Part print with two shaded views. Sizes in mm from the minimum x, y, z corner. A direction names the side the tool comes from. Round coordinates to 2 decimals unless told otherwise and drop trailing zeros. Write each loop counter-clockwise with the first axis right and the second up, starting at its lowest first coordinate (ties: lowest second). Pieces come first, ordered by that corner, then holes. Notation, with made-up numbers: (22.5, 2.5) -> (72.5, 2.5) arc R25 ccw to (72.5, 29.5) -> close; hole circle Ø2 at (-29, 22). An arc over 180 degrees is marked (long way). Return JSON: item names as keys, results as strings. Group by question number.
(1) Drill centre lines: L1, parallel to Y at x = 20, z = 11.7; L2, parallel to X at y = 8.75, z = 15; L3, parallel to Z at x = 18, y = 19. Where is each one in solid material? Low to high. Write a range as from..to.
(2) Drop flat-ended pins along their axis: pin 1 Ø6.5 at (x, y) = (20, 12.5) entering from +Z; pin 2 Ø13 at (x, y) = (18.5, 14.5) entering from +Z; pin 3 Ø10 at (x, z) = (8.5, 7) entering from +Y; pin 4 Ø8 at (x, y) = (20, 0.5) entering from -Z. Give the stop position or say it passes through.
(3) Mould opens along X. For the marked faces 5, 6, 7 and 8 say: +X half, -X half, draft (parallel to the pull), parting line (faces both ways), or undercut.
(4) Saw through at A-A (z = 8.5). List the corners of the cut face in (x, y), plus the area to 3 significant figures.
(5) Saw through at D-D (y = 8.75). List the corners of the cut face in (x, z), plus the area to 4 significant figures.
(6) Tool access for the marked faces 1, 2, 3 and 4: list every direction of +Z, -Z, +X, -X, +Y, -Y with a clear straight run to the whole face (end or side of a thin tool).
(7) Saw through at B-B (x = 20). List the corners of the cut face in (y, z).
(8) Saw through at C-C (y = 2.5). List the corners of the cut face in (x, z), plus the area to 4 significant figures.
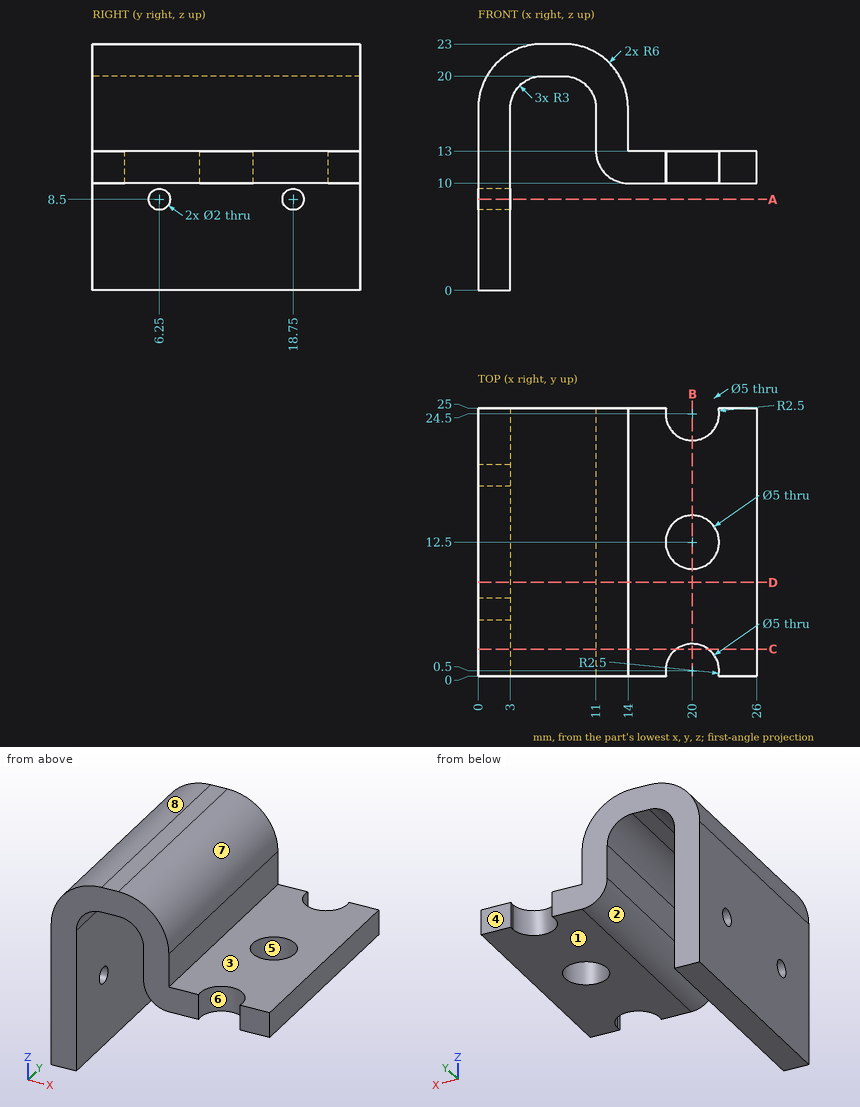
Computed values:
{
 "1": {"L1": "3..10, 15..22", "L2": "0..3, 11..14", "L3": "10..13"},
 "2": {"pin 1": "z = 13", "pin 2": "z = 21.47", "pin 3": "through", "pin 4": "z = 10"},
 "3": {"face 5": "undercut", "face 6": "undercut", "face 7": "+X half", "face 8": "-X half"},
 "4": {"outline": "(0, 0) -> (3, 0) -> (3, 5.25) -> (0, 5.25) -> close; (0, 7.25) -> (3, 7.25) -> (3, 17.75) -> (0, 17.75) -> close; (0, 19.75) -> (3, 19.75) -> (3, 25) -> (0, 25) -> close", "area": "63.0 mm2"},
 "5": {"outline": "(0, 0) -> (3, 0) -> (3, 17) arc R3 cw to (6, 20) -> (8, 20) arc R3 cw to (11, 17) -> (11, 13) arc R3 ccw to (14, 10) -> (26, 10) -> (26, 13) -> (14, 13) -> (14, 17) arc R6 ccw to (8, 23) -> (6, 23) arc R6 ccw to (0, 17) -> close", "area": "154.5 mm2"},
 "6": {"face 1": "-Z, +X, +Y, -Y", "face 2": "-Z, +Y, -Y", "face 3": "+Z, +X, +Y, -Y", "face 4": "+Z, -Z, +X, -X, +Y"},
 "7": {"outline": "(3, 10) -> (10, 10) -> (10, 13) -> (3, 13) -> close; (15, 10) -> (22, 10) -> (22, 13) -> (15, 13) -> close"},
 "8": {"outline": "(0, 0) -> (3, 0) -> (3, 17) arc R3 cw to (6, 20) -> (8, 20) arc R3 cw to (11, 17) -> (11, 13) arc R3 ccw to (14, 10) -> (18.5, 10) -> (18.5, 13) -> (14, 13) -> (14, 17) arc R6 ccw to (8, 23) -> (6, 23) arc R6 ccw to (0, 17) -> close; (21.5, 10) -> (26, 10) -> (26, 13) -> (21.5, 13) -> close", "area": "145.5 mm2"}
}
